Autodesk Inventor part; units mm, degrees
ref_plane "YZ Plane" through (0, 0, 0) normal (1, 0, 0) x (0, 1, 0)
ref_plane "XZ Plane" through (0, 0, 0) normal (0, 1, 0) x (-1, 0, 0)
ref_plane "XY Plane" through (0, 0, 0) normal (0, 0, 1) x (1, 0, 0)
sketch "Sketch1" plane through (0, 0, 0) normal (0, 0, 1) x (1, 0, 0)
  arc A0 (50.165, -86.8883) -> (-50.165, -86.8883) centre (0, 0) ccw
  line L0 (0, 123.825) -> (0, 0) construction
  line L1 (-168.8677, 119.38) -> (168.8677, 119.38) construction
  line L2 (127, 119.38) -> (127, -44.6491)
  line L3 (0, 0) -> (67.31, -116.5843) construction
  line L4 (50.165, -86.8883) -> (67.31, -116.5843)
  line L5 (-127, 119.38) -> (-127, -44.6491)
  line L6 (0, 0) -> (-67.31, -116.5843) construction
  line L7 (-50.165, -86.8883) -> (-67.31, -116.5843)
  arc A1 (-50.165, 325.6483) -> (50.165, 325.6483) centre (0, 238.76) ccw
  line L8 (127, 119.38) -> (127, 283.4091)
  line L9 (50.165, 325.6483) -> (67.31, 355.3443)
  line L10 (-127, 119.38) -> (-127, 283.4091)
  line L11 (-50.165, 325.6483) -> (-67.31, 355.3443)
  arc A2 (127, 283.4091) -> (67.31, 355.3443) centre (0, 238.76) ccw
  arc A3 (-67.31, 355.3443) -> (-127, 283.4091) centre (0, 238.76) ccw
  arc A4 (-127, -44.6491) -> (-67.31, -116.5843) centre (0, 0) ccw
  arc A5 (67.31, -116.5843) -> (127, -44.6491) centre (0, 0) ccw
  point P0 (114.3, -45.72)
  point P1 (0, 119.38)
  point P2 (-114.3, -45.72)
  point P3 (114.3, 284.48)
  point P4 (-114.3, 284.48)
  dimension "d1" = 200.66
  dimension "d18" = 119.38
  dimension "d19" = 165.1
  dimension "d20" = 114.3
  dimension "d25" = 127
  dimension "d26" = 150
  dimension "d34" = 134.62
extrude "Extrusion1" add sketch "Sketch1" along normal blind 6.35
hole "Hole2" at (114.3, -45.72, 0) at (0, 119.38, 0) at (-114.3, -45.72, 0) at (114.3, 284.48, 0) at (-114.3, 284.48, 0) direction (0, 0, 1) diameter 6.7564 end through all
fillet "Fillet1" radius 6.35 8 edges at (50.165, -86.8883, 3.175) (-50.165, -86.8883, 3.175) (67.31, 355.3443, 3.175) (-67.31, 355.3443, 3.175) (50.165, 325.6483, 3.175) (-50.165, 325.6483, 3.175) (67.31, -116.5843, 3.175) (-67.31, -116.5843, 3.175)
properties part number "J001393" material "ALUMINUM, 6061-T651"
Source: CAD feature listing. Evaluate the final solid. Frame: model axes, mm. A direction names the side the tool comes from. Round coordinates to 2 decimals unless told otherwise and drop trailing zeros. Order: outer loops, then holes, each group sorted by start corner. A loop starts at its lowest first (then second) coordinate and runs counter-clockwise, first axis right, second up. Notation, with made-up numbers: (-30.5, 88.25) - (24.5, 88.25) arc R14 ccw to (24.5, 100.25) - close; hole circle Ø6 at (-38, 80.25). An arc over 180 degrees is marked (long way). Use a Markdown table: item, result. Add a question column.
1. Line query: probe 1 along Y at (x, z) = (70.5, 0.5); probe 2 along Y at (x, z) = (-69, 2); probe 3 along X at (y, z) = (284.48, 3.5). Output: solid intervals per line, ascending.
2. Set-up query: faces 5 (the flat face through (-58.6, -101.5, 3.1)), 6 (the cylindrical face through (106.08, -82.88, 3.13)), 7 (the flat face through (58.58, 340.22, 3.13)). Return all of +Z, -Z, +X, -X, +Y, -Y with unobstructed straight access to the full face (end or side cutting, diameter ignored); none if empty.
3. Section query C-C (y = -78). Return the cut outline in (x, z), then the cut area to 3 significant figures.
4. Section query D-D (x = -29). Return the cut outline in (y, z).
5. Section query A-A (y = 238.76). Return the cut outline in (x, z), then the cut area to 3 significant figures.
6. Mould query, pull axis X, two halves, no side actions, for faces 1 (the flat face through (-58.58, 340.22, 3.13)), 2 (the cylindrical face through (-106.08, 321.64, 3.13)), 3 (the flat face through (58.6, -101.5, 3.1)), 4 (the flat face through (-2, 123, 0)). Classes: +X half, -X half, draft (parallel to the pull), parting line (faces both ways), or undercut.
7. First-contact query: pin 1 (4 mm diameter, centred on x = 114.3, y = 284.48, fed in from +Z). Flat tip, straight axial feed; report the tip coordinate or a pass-through.
8. Section query B-B (z = 3.5). Return the cut outline in (x, y).
Derived:
| question | item | result |
|---|---|---|
| 1 | probe 1 | -114.05 to -71.39, 71.39 to 167.37, 310.15 to 352.81 |
| 1 | probe 2 | -114.1 to -72.84, 72.84 to 165.92, 311.6 to 352.86 |
| 1 | probe 3 | -126.62 to -117.68, -110.92 to -89.31, 89.31 to 110.92, 117.68 to 126.62 |
| 2 | face 5 | +Z, -Z, -Y |
| 2 | face 6 | +Z, -Z, +X, -Y |
| 2 | face 7 | +Z, -Z, +Y |
| 3 | outline | (-109.72, 0) - (-63.1, 0) - (-63.1, 6.35) - (-109.72, 6.35) - close; (63.1, 0) - (109.72, 0) - (109.72, 6.35) - (63.1, 6.35) - close |
| 3 | area | 592 mm2 |
| 4 | outline | (96.05, 0) - (142.71, 0) - (142.71, 6.35) - (96.05, 6.35) - close |
| 5 | outline | (-127, 0) - (-100.33, 0) - (-100.33, 6.35) - (-127, 6.35) - close; (100.33, 0) - (127, 0) - (127, 6.35) - (100.33, 6.35) - close |
| 5 | area | 339 mm2 |
| 6 | face 1 | undercut |
| 6 | face 2 | -X half |
| 6 | face 3 | undercut |
| 6 | face 4 | draft |
| 7 | pin 1 | through |
| 8 | outline | (-127, -44.65) arc R134.62 ccw to (-73, -113.11) arc R6.35 ccw to (-64.06, -110.95) - (-53.25, -92.22) arc R6.35 ccw to (-55.25, -83.75) arc R100.33 cw (long way) to (55.25, -83.75) arc R6.35 ccw to (53.25, -92.22) - (64.06, -110.95) arc R6.35 ccw to (73, -113.11) arc R134.62 ccw to (127, -44.65) - (127, 283.41) arc R134.62 ccw to (73, 351.87) arc R6.35 ccw to (64.06, 349.71) - (53.25, 330.98) arc R6.35 ccw to (55.25, 322.51) arc R100.33 cw (long way) to (-55.25, 322.51) arc R6.35 ccw to (-53.25, 330.98) - (-64.06, 349.71) arc R6.35 ccw to (-73, 351.87) arc R134.62 ccw to (-127, 283.41) - close; hole circle Ø6.76 at (-114.3, -45.72); hole circle Ø6.76 at (-114.3, 284.48); hole circle Ø6.76 at (0, 119.38); hole circle Ø6.76 at (114.3, -45.72); hole circle Ø6.76 at (114.3, 284.48) |
